Could you check a few things on this model? Use its own coordinates, in mm. Face numbers are marked on the shaded views. A direction names the side the tool comes from. Give positions to 0.01 mm unless a question says otherwise; leave off trailing zeros. Loops run counter-clockwise (first coordinate to the right, second up) from the corner with the lowest first, then second, coordinate; pieces in that order, holes last.
1. For the marked faces 1, 2, 3 and 4, which set-ups out of +Z, -Z, +X, -X, +Y, -Y let a thin tool reach every point of the face, with its end or its side?
2. Imagine slicing it at C-C (y = -1.75). List the corners of the cut face in (x, z) for me.
3. Imagine slicing it at B-B (z = -7.5). List the corners of the cut face in (x, y) for me, plus the area to 3 significant figures.
4. For P1, Ø5, axis at x = -56.5, y = -1.5, coming from the -Z side; P2, Ø0.6, axis at y = -3, z = 2, coming from the -X side; P3, Ø2.5, axis at x = -57, y = -0.5, coming from the -Z side; P4, Ø1.3, axis at y = -1, z = -3, coming from the -X side, each with a flat end and sliding along its axis, tell me the tip position at first contact or that it passes through.
5. Imagine slicing it at A-A (x = -54.2). List the corners of the cut face in (y, z) for me.
6. I need wall thicknesses on line 1 along X through (y, z) = (0, -2.5); line 2 along Y through (x, z) = (-54.5, 0.75); line 3 along Z through (x, y) = (-60.5, -0.75). Which ranges of each line are inside material? Lowest first, please.
7. Imagine slicing it at D-D (y = 0.5). List the corners of the cut face in (x, z) for me.
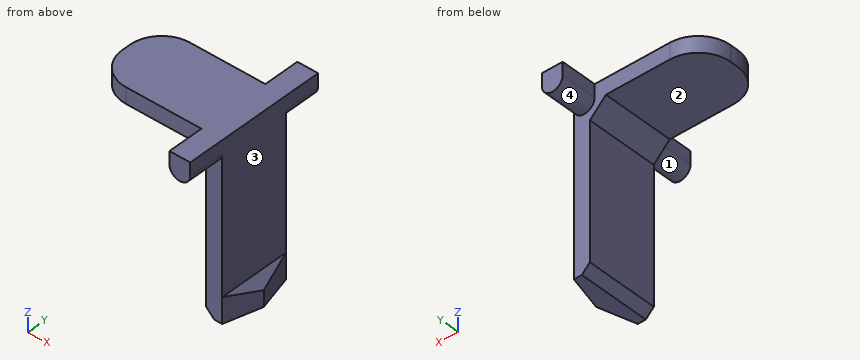
```python
from build123d import *

# Parameters (mm, degrees)
PAD003_DEPTH         = 2.25
PAD004_DEPTH         = 4.5
POCKET013_DEPTH      = 33.508955
POCKET013_DEPTH_BACK = 43.758955
FILLET_R             = 2


with BuildPart() as part:
    # Sketch027 → Pad003 (new body, symmetric)
    with BuildSketch(Plane.XZ):
        Polygon((-61.55, 1.6), (-55.55, 1.6), (-54.55, 0.6), (-54.55, -7.85), (-54.05, -8.35), (-52.95, -8.35), (-52.95, -7.35), (-53.55, -6.75), (-53.55, 2.6), (-61.55, 2.6), align=None)
    extrude(amount=PAD003_DEPTH, both=True)

    # Sketch028 → Pad004 (join, symmetric)
    with BuildSketch(Plane.XZ):
        with BuildLine():
            ThreePointArc((-54.85, 1.8), (-54.2, 1.15), (-53.55, 1.8))
            Line((-53.55, 1.8), (-53.55, 2.6))
            Line((-53.55, 2.6), (-54.85, 2.6))
            Line((-54.85, 1.8), (-54.85, 2.6))
        make_face()
    extrude(amount=PAD004_DEPTH, both=True)

    # Sketch029 (on DatumPlane) → Pocket013 (cut, two sides)
    with BuildSketch(Plane.XY.offset(-8)) as pocket013_sk:
        Polygon((-52.95, 2.25), (-53.55, 2.25), (-52.95, 0), align=None)
    pocket013 = extrude(amount=-POCKET013_DEPTH, mode=Mode.SUBTRACT) + extrude(pocket013_sk.sketch, amount=POCKET013_DEPTH_BACK, mode=Mode.SUBTRACT)

    # Mirrored001: Pocket013 across XZ
    add(pocket013.mirror(Plane.XZ), mode=Mode.SUBTRACT)

    # Fillet
    fillet_edges = [part.edges().sort_by_distance(p)[0] for p in [
        (-61.55, 2.25, 2.1),
        (-61.55, -2.25, 2.1),
    ]]
    fillet(fillet_edges, radius=FILLET_R)


solid = part.part
```
Derived:
1. face 1: -Z, -Y
1. face 2: -Z, -X, +Y, -Y
1. face 3: +Z, +X, +Y, -Y
1. face 4: -Z, +Y
2. outline: (-60.87, 1.6) - (-55.55, 1.6) - (-54.55, 0.6) - (-54.55, -7.85) - (-54.05, -8.35) - (-53.42, -8.35) - (-53.42, -6.88) - (-53.55, -6.75) - (-53.55, 2.6) - (-60.87, 2.6) - close
3. outline: (-54.55, -2.25) - (-53.55, -2.25) - (-52.95, 0) - (-53.55, 2.25) - (-54.55, 2.25) - close
3. area: 5.85 mm2
4. P1: stops at z = -8.35
4. P2: stops at x = -54.85
4. P3: stops at z = 1.6
4. P4: stops at x = -54.55
5. outline: (-4.5, 1.15) - (-2.25, 1.15) - (-2.25, -8.2) - (2.25, -8.2) - (2.25, 1.15) - (4.5, 1.15) - (4.5, 2.6) - (-4.5, 2.6) - close
6. line 1: x = -54.55 to -53.55
6. line 2: y = -2.25 to 2.25
6. line 3: z = 1.6 to 2.6
7. outline: (-61.53, 1.6) - (-55.55, 1.6) - (-54.55, 0.6) - (-54.55, -7.85) - (-54.05, -8.35) - (-53.08, -8.35) - (-53.08, -7.22) - (-53.55, -6.75) - (-53.55, 2.6) - (-61.53, 2.6) - close
